```python
from build123d import *

# Parameters (mm, degrees)
SKETCH2_R               = 4.75
BOSS_EXTRUDE1_DEPTH     = 77
SKETCH4_R               = 4.125
CUT_EXTRUDE1_DEPTH      = 77
CUT_EXTRUDE2_DEPTH      = 77
CUT_EXTRUDE3_DEPTH      = 77
CUT_EXTRUDE3_DEPTH_BACK = 77
BOSS_EXTRUDE2_START     = 4
BOSS_EXTRUDE2_DEPTH     = 4
CHAMFER1_SIZE           = 6
CHAMFER1_SIZE_2         = 3.5


with BuildPart() as part:
    # Sweep1: sweep along a path in Sketch1
    with BuildLine(Plane.XY) as sweep1_path:
        Line((0, 0), (940, 0))
        Line((940, 0), (960, 16.781992624))
        Line((960, 16.781992624), (1016, 16.781992624))
    # Sketch2 → Sweep1 (sweep)
    with BuildSketch(Plane(origin=(0, 0, 0), x_dir=(0, 0, -1), z_dir=(1, 0, 0))):
        Circle(SKETCH2_R)
    sweep(path=sweep1_path.line, transition=Transition.RIGHT)

    # Sketch3 → Boss-Extrude1 (add)
    with BuildSketch(Plane(origin=(1016, 0, 0), x_dir=(0, 0, -1), z_dir=(1, 0, 0))):
        with BuildLine():
            Line((-7.071067812, 12.031992624), (7.071067812, 12.031992624))
            ThreePointArc((7.071067812, 12.031992624), (7.5, 14.531992624), (7.071067812, 17.031992624))
            Line((7.071067812, 17.031992624), (-7.071067812, 17.031992624))
            ThreePointArc((-7.071067812, 17.031992624), (-7.5, 14.531992624), (-7.071067812, 12.031992624))
        make_face()
    extrude(amount=BOSS_EXTRUDE1_DEPTH)

    # Sketch4 → Cut-Extrude1 (cut)
    with BuildSketch(Plane(origin=(0, 17.031992624, 0), x_dir=(1, 0, 0), z_dir=(0, 1, 0))):
        with Locations(Location((1084.475, 0, 0), (0, 0, 270))):
            Circle(SKETCH4_R)
    extrude(amount=-CUT_EXTRUDE1_DEPTH, mode=Mode.SUBTRACT)

    # Sketch5 → Cut-Extrude2 (cut)
    with BuildSketch(Plane(origin=(0, 17.031992624, 0), x_dir=(1, 0, 0), z_dir=(0, 1, 0))):
        with BuildLine():
            Line((1093, 7.5), (1088.527853933, 7.5))
            ThreePointArc((1088.527853933, 7.5), (1093, 0), (1088.527853933, -7.5))
            Line((1088.527853933, -7.5), (1093, -7.5))
            Line((1093, -7.5), (1095.488265068, 1.431081092))
            Line((1095.488265068, 1.431081092), (1093, 7.5))
        make_face()
    extrude(amount=-CUT_EXTRUDE2_DEPTH, mode=Mode.SUBTRACT)

    # Sketch6 → Cut-Extrude3 (cut, two sides: drawn at the far end of the back side and taken through both)
    with BuildSketch(Plane.XY.offset(-CUT_EXTRUDE3_DEPTH_BACK)):
        Polygon((1016, 17.031992624), (1012, 21.531992624), (1018.885341188, 26.165219669), (1022.40477818, 20.935058436), align=None)
    extrude(amount=CUT_EXTRUDE3_DEPTH + CUT_EXTRUDE3_DEPTH_BACK, mode=Mode.SUBTRACT)

    # Sketch7 → Boss-Extrude2 (add)
    with BuildSketch(Plane.ZY.offset(-1016).offset(BOSS_EXTRUDE2_START)):
        with BuildLine():
            Line((7.071067812, 17.031992624), (4.74341649, 17.031992624))
            Line((4.74341649, 17.031992624), (-4.74341649, 17.031992624))
            Line((-4.74341649, 17.031992624), (-7.071067812, 17.031992624))
            ThreePointArc((-7.071067812, 17.031992624), (-7.5, 14.531992624), (-7.071067812, 12.031992624))
            Line((-7.071067812, 12.031992624), (0, 12.031992624))
            Line((0, 12.031992624), (7.071067812, 12.031992624))
            ThreePointArc((7.071067812, 12.031992624), (7.5, 14.531992624), (7.071067812, 17.031992624))
        make_face()
    extrude(amount=-BOSS_EXTRUDE2_DEPTH)

    # Chamfer1
    # the kernel refuses this chamfer: 6, 3.5 mm, written as the material it takes off along each edge
    with BuildSketch(Plane(origin=(1012, 14.531992624, 0), x_dir=(0, 0.6684369034983231, 0.7437688525621206), z_dir=(0, -0.7437688525621206, 0.6684369034983231))) as chamfer1_piece_1_section:
        Polygon((7.5, -CHAMFER1_SIZE), (7.5 - CHAMFER1_SIZE_2, 0), (7.5, 0), align=None)
    chamfer1_piece_1 = revolve(axis=Axis((1012, 14.531992624, 0), (-1, 0, 0)), revolution_arc=276.106922799, mode=Mode.PRIVATE)
    chamfer1_piece_1 = chamfer1_piece_1 - Plane(origin=(1014.966337757, 16.781992624, 0), x_dir=(0, 0, -1), z_dir=(1, 0, 0)) * Cylinder(4.75, 30, mode=Mode.PRIVATE)
    add(chamfer1_piece_1, mode=Mode.SUBTRACT)
    with BuildSketch(Plane(origin=(1012, 14.531992624, 0), x_dir=(0, -0.668436903498336, -0.743768852562109), z_dir=(0, 0.743768852562109, -0.668436903498336))) as chamfer1_piece_2_section:
        Polygon((7.5 - CHAMFER1_SIZE_2, 0), (7.5, -CHAMFER1_SIZE), (7.5, 0), align=None)
    chamfer1_piece_2 = revolve(axis=Axis((1012, 14.531992624, 0), (-1, 0, 0)), revolution_arc=276.106922799, mode=Mode.PRIVATE)
    chamfer1_piece_2 = chamfer1_piece_2 - Plane(origin=(1014.966337768, 16.781992624, 0), x_dir=(0, 0, -1), z_dir=(1, 0, 0)) * Cylinder(4.75, 31, mode=Mode.PRIVATE)
    add(chamfer1_piece_2, mode=Mode.SUBTRACT)


solid = part.part
```
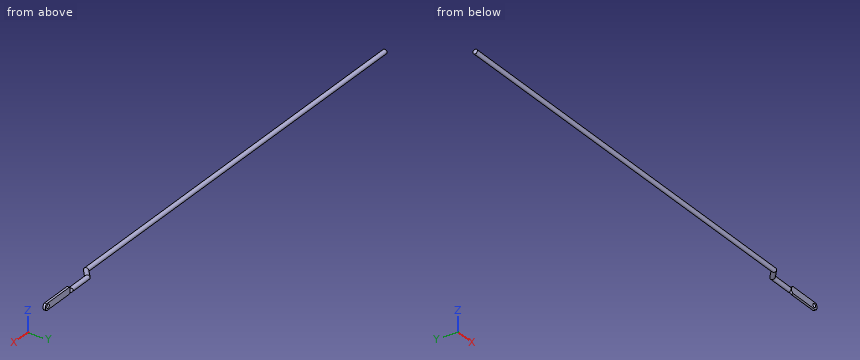
Design review of the part built by this model. Coordinates are the model's own, in mm. Give positions to 0.01 mm unless a question says otherwise; leave off trailing zeros. Write each loop counter-clockwise with the first axis right and the second up, starting at its lowest first coordinate (ties: lowest second). Pieces come first, ordered by that corner, then holes. Notation, with made-up numbers: (19, 35) - (70, 35) arc R26 cw to (70, 65) - close; hole circle Ø1 at (79.25, 35.5). An arc over 180 degrees is marked (long way). Return JSON: item names as keys, results as strings. Group by question number.
(1) To check wall thickness, follow probe 1 along Z at (x, y) = (410.5, -3.5); probe 2 along X at (y, z) = (13.65, 0). State the ranges of each line that lie inside material, in increasing order.
(2) We need section A-A, the plane x = 811. Give the boundary of the cut face in (y, z), then the cut area to 3 significant figures.
(3) Insertion check: pin 1 (3 mm diameter, centred on x = 127, z = 2, fed in from +Y); pin 2 (8 mm diameter, centred on y = 14.5, z = -6, fed in from +X); pin 3 (2 mm diameter, centred on y = 8.5, z = 3.5, fed in from +X); pin 4 (8 mm diameter, centred on y = 2, z = -2, fed in from -X). Each pin has a flat end and moves straight along its axis. Give the tip position at first contact, or say it passes through.
Reported:
{
 "1": {"probe 1": "z = -3.21 to 3.21", "probe 2": "x = 948.88 to 1080.35, 1088.6 to 1093"},
 "2": {"outline": "circle Ø9.5 at (0, 0)", "area": "70.9 mm2"},
 "3": {"pin 1": "stops at y = 4.72", "pin 2": "stops at x = 1092.76", "pin 3": "stops at x = 956.95", "pin 4": "stops at x = 0"}
}
